Autodesk Inventor part; units mm, degrees
ref_plane "YZ Plane" through (0, 0, 0) normal (1, 0, 0) x (0, 1, 0)
ref_plane "XZ Plane" through (0, 0, 0) normal (0, 1, 0) x (-1, 0, 0)
ref_plane "XY Plane" through (0, 0, 0) normal (0, 0, 1) x (1, 0, 0)
sketch "Эскиз1" plane through (0, 0, 0) normal (1, 0, 0) x (0, 1, 0)
  line L0 (0, 0) -> (13.9611, 0) construction
  line L1 (0, 26.35) -> (-10, 26.35) construction
  line L2 (-10, 26.35) -> (-10, -26.35) construction
  line L3 (-10, -26.35) -> (0, -26.35) construction
  line L4 (0, -26.35) -> (0, 26.35) construction
  line L5 (0, 0) -> (0, -22.0675) construction
  line L6 (2, 25) -> (0, 25) construction
  line L7 (0, 25) -> (0, -25) construction
  line L8 (0, -25) -> (2, -25) construction
  line L9 (2, -25) -> (2, 25) construction
  line L10 (5, -19) -> (5, -30.35)
  line L11 (-2, -11.433) -> (-2, -38.2242) construction
  line L12 (5, -19) -> (2, -19)
  line L13 (5, -30.35) -> (2, -30.35)
  line L14 (2, -30.35) -> (2, -19)
  dimension "d0" = 10
  dimension "d1" = 52.7
  dimension "d2" = 2
  dimension "d3" = 50
  dimension "d4" = 3
  dimension "d6" = 2
  dimension "d7" = 6
  dimension "d8" = 3
  dimension "d10" = 4
revolve "Вращение1" add sketch "Эскиз1" angle 360 about axis through (0, 0, 0) along (0, 1, 0)
chamfer "Фаска1" distance 1.5 angle 55 1 edges at (0, 5, 19) measured on face at (2.4211, 5, -26.2727)
sketch "Эскиз2" plane through (0, 0, 0) normal (0, 0, 1) x (1, 0, 0)
  line L0 (-30.35, 5) -> (30.35, 5) construction
  line L1 (-30.35, 2) -> (30.35, 2) construction
  line L2 (-19, 2.8578) -> (19, 2.8578) construction
  line L3 (20.5, 5) -> (-20.5, 5) construction
  line L4 (-19, 2) -> (19, 2) construction
  line L5 (-19, 2.8578) -> (19, 2.8578) construction
  line L6 (0, 0) -> (25, 0) construction
  line L7 (25, 2) -> (25, -8.0068) construction
  line L8 (-30.35, 2) -> (30.35, 2) construction
  line L9 (25.2, 2) -> (25.2, -4.9803) construction
  line L10 (25.45, 1.5) -> (25.45, 1.5) construction
  line L11 (26.2, 1.5) -> (26.2, 0) construction
  line L12 (26.2, 0) -> (25.45, 0) construction
  line L13 (24.7, 0.75) -> (24.7, 0.75) construction
  line L14 (26.2, 0) -> (26.2, 0) construction
  line L15 (28.2, 2) -> (28.2, 2) construction
  line L16 (28.2, 2) -> (26.2, 2) construction
  line L17 (26.2, 2) -> (26.2, 2.25) construction
  arc A0 (25.45, 1.5) -> (24.7, 0.75) centre (25.45, 0.75) ccw
  arc A1 (24.7, 0.75) -> (25.45, 0) centre (25.45, 0.75) ccw
  arc A2 (26.2, 0) -> (28.2, 2) centre (26.2, 2) ccw
  line L18 (25.95, 2) -> (28.2, 2)
  line L19 (25.45, 0) -> (26.2, 0)
  line L20 (-19, 2) -> (19, 2)
  line L21 (0, 2) -> (0, 5)
  line L22 (-30.35, 5) -> (30.35, 5)
  line L23 (25.45, 1.5) -> (25.95, 2)
  point P0 (24.7, 0)
  point P1 (24.7, 0.75)
  point P2 (25.45, 1.5)
  dimension "d15" = 25
  dimension "d16" = 0.2
  dimension "d17" = 1.5
  dimension "d18" = 1.5
  dimension "d19" = 0.5
  dimension "d20" = 2
  dimension "d21" = 0.75
  dimension "d22" = 2
  dimension "d31" = 45
revolve "Вращение2" add sketch "Эскиз2" angle 45 mid plane about axis through (0, 2, 0) along (0, 1, 0)
pattern_circular "Круговой массив1" count 4 over 360 about axis through (0, 3.5, 0) along (0, -1, 0) of "Вращение2"
sketch "Эскиз3" plane through (0, 0, 0) normal (0, 0, 1) x (1, 0, 0)
  line L0 (-30.35, 5) -> (30.35, 5) construction
  line L1 (20.5, 5) -> (-20.5, 5) construction
  arc A0 (-28.2, 2) -> (-26.2, 0) centre (-26.2, 2) ccw construction
  line L2 (-28.2, 2) -> (-28.2, 5)
  line L3 (-28.2, 5) -> (-20.5, 5) construction
  line L4 (-28.2, 2) -> (-31.4016, 2)
  line L5 (-31.4016, 2) -> (-31.4016, 5.1774)
  line L6 (-31.4016, 5.1774) -> (-28.2, 5.1774)
  line L7 (-28.2, 5.1774) -> (-28.2, 2)
  line L8 (0, 0) -> (0, 5)
revolve "Вращение3" cut sketch "Эскиз3" angle 360 about axis through (0, 0, 0) along (0, 1, 0)
chamfer "Фаска2" distance 1.5 angle 55 1 edges at (28.2, 5, 0) measured on face at (-25.3104, 5, -3.0732)
properties part number "mirror_lock_v1"
Input: part model. Units: mm. Frame: model coordinates. A direction names the side the tool comes from. Give positions to 0.01 mm unless a question says otherwise; leave off trailing zeros. Loops run counter-clockwise (first coordinate to the right, second up) from the corner with the lowest first, then second, coordinate; pieces in that order, holes last. Notation, with made-up numbers: (33.5, -12.5) -> (92.5, -12.5) arc R15 ccw to (92.5, 15.5) -> close; hole circle Ø7 at (-12, 16). An arc over 180 degrees is marked (long way). Answer as a JSON object with one key per item and string values. Group by question number.
Item 1: Pin query (flat end, axial travel): P1, Ø4, axis at x = -13, z = -20.5, coming from the -Y side. Return the tip coordinate at first contact, or that it passes through.
Item 2: Line query: probe 1 along Z at (x, y) = (0, 2.3); probe 2 along Y at (x, z) = (-21, 8). Output: solid intervals per line, ascending.
Item 3: Pull-direction query (Y, two-part tool) for faces 4 (the flat face through (-26, 0, 0)), 5 (the conical face through (0.14, 1.64, -25.59)), 6 (the conical face through (5.808, 4.866, 26.157)); classes: released by +Y, released by -Y, zero draft, split by the parting line, or undercut.
Item 4: Cut plane A-A, the plane z = 0. Return the cut outline in (x, y), and give its area (3 significant figures).
Item 5: Cut plane B-B, the plane x = 0. Return the cut outline in (y, z).
Item 6: Reachability of faces 1 (the conical face through (-25.59, 1.64, -0.14)), 2 (the flat face through (24.41, 1.01, -10.11)), 3 (the flat face through (24.41, 1.01, 10.11)) from +Z, -Z, +X, -X, +Y, -Y: full face, straight path, thin tool, end or side. Return the list, or none.
Checks:
{
 "1": {"P1": "stops at y = 2"},
 "2": {"probe 1": "z = -28.2 to -19, 19 to 28.2", "probe 2": "y = 2 to 5"},
 "3": {"face 4": "released by -Y", "face 5": "undercut", "face 6": "released by +Y"},
 "4": {"outline": "(-28.2, 2) arc R2 ccw to (-26.2, 0) -> (-25.45, 0) arc R0.75 ccw to (-25.45, 1.5) -> (-25.95, 2) -> (-19, 2) -> (-19, 2.86) -> (-20.5, 5) -> (-26.7, 5) -> (-28.2, 2.86) -> close; (19, 2) -> (25.95, 2) -> (25.45, 1.5) arc R0.75 ccw to (25.45, 0) -> (26.2, 0) arc R2 ccw to (28.2, 2) -> (28.2, 2.86) -> (26.7, 5) -> (20.5, 5) -> (19, 2.86) -> close", "area": "59.6 mm²"},
 "5": {"outline": "(0, -26.2) arc R2 ccw to (2, -28.2) -> (2.86, -28.2) -> (5, -26.7) -> (5, -20.5) -> (2.86, -19) -> (2, -19) -> (2, -25.95) -> (1.5, -25.45) arc R0.75 ccw to (0, -25.45) -> close; (0, 25.45) arc R0.75 ccw to (1.5, 25.45) -> (2, 25.95) -> (2, 19) -> (2.86, 19) -> (5, 20.5) -> (5, 26.7) -> (2.86, 28.2) -> (2, 28.2) arc R2 ccw to (0, 26.2) -> close"},
 "6": {"face 1": "none", "face 2": "-Z, -Y", "face 3": "+Z, -Y"}
}
